from build123d import *

# Parameters (mm, degrees)
F0_W     = 20
F0_H     = 12
F1_DEPTH = 6
F2_R     = 1.6175230868
F4_DEPTH = 0.3
F5_W     = 9.6640973352
F5_H     = 2.0774973091
F6_DEPTH = 0.1
F8_DEPTH = 25


with BuildPart() as f1:
    # F0 (on Top) → F1 (new body)
    with BuildSketch(Plane.XY):
        Rectangle(F0_W, F0_H)
    extrude(amount=F1_DEPTH)

    # F2
    f2_edges = [f1.edges().sort_by_distance(p)[0] for p in [
        (10, 0, 6),
        (-10, 0, 6),
    ]]
    fillet(f2_edges, radius=F2_R)

    # F3 (on face) → F4 (join)
    with BuildSketch(Plane(origin=(0, 6, 0), x_dir=(-1, 0, 0), z_dir=(0, 1, 0))):
        with BuildLine():
            add(Edge.make_bspline(
                [(-5.9889552958, 4.3307738066), (-6.7707574457, 5.2428768765), (-7.1497281936, 4.126935614), (-7.5286989414, 3.0109943515), (-6.3679260436, 3.2148325442), (-5.2071531458, 3.4186707368), (-5.9889552958, 4.3307738066)],
                knots=[4.7123889804, 4.7123889804, 4.7123889804, 6.8067840828, 6.8067840828, 8.9011791852, 8.9011791852, 10.9955742876, 10.9955742876, 10.9955742876], degree=2, weights=[1, 0.5, 1, 0.5, 1, 0.5, 1]))
        make_face()
        Polygon((-7.1114664897, 3.8173154462), (-6.1345444992, 4.4055692852), (-6.2445141857, 3.376125358), align=None, mode=Mode.SUBTRACT)
        with BuildLine():
            add(Edge.make_bspline(
                [(5.9889552958, 4.3307738066), (5.2071531458, 3.4186707368), (6.3679260436, 3.2148325442), (7.5286989414, 3.0109943515), (7.1497281936, 4.126935614), (6.7707574457, 5.2428768765), (5.9889552958, 4.3307738066)],
                knots=[4.7123889804, 4.7123889804, 4.7123889804, 6.8067840828, 6.8067840828, 8.9011791852, 8.9011791852, 10.9955742876, 10.9955742876, 10.9955742876], degree=2, weights=[1, 0.5, 1, 0.5, 1, 0.5, 1]))
        make_face()
        Polygon((6.1345444992, 4.4055692852), (7.1114664897, 3.8173154462), (6.2445141857, 3.376125358), align=None, mode=Mode.SUBTRACT)
    extrude(amount=F4_DEPTH)

    # F5 (on face) → F6 (join)
    with BuildSketch(Plane(origin=(0, 6, 0), x_dir=(-1, 0, 0), z_dir=(0, 1, 0))):
        with Locations((-0.4735698458, 1.9353075186)):
            Rectangle(F5_W, F5_H)
        Polygon((-5.069738923, 1.1018711375), (-5.069738923, 2.8125192574), (-4.8855133355, 2.8125192574), (-3.3977353226, 2.8125192574), (-3.2135097351, 2.8125192574), (-1.7257317222, 2.8125192574), (-1.5415061347, 2.8125192574), (-0.0537281219, 2.8125192574), (0.1304974656, 2.8125192574), (1.6182754785, 2.8125192574), (1.802501066, 2.8125192574), (3.2902790789, 2.8125192574), (3.4745046664, 2.8125192574), (4.1262808791, 2.8125192574), (4.1262808791, 1.4788382144), (4.1262808791, 1.1018711375), (2.6385028662, 1.1018711375), (2.4542772787, 1.1018711375), (0.9664992658, 1.1018711375), (0.7822736783, 1.1018711375), (-0.7055043345, 1.1018711375), (-0.889729922, 1.1018711375), (-2.3775079349, 1.1018711375), (-2.5617335224, 1.1018711375), (-4.0495115353, 1.1018711375), (-4.2337371228, 1.1018711375), align=None, mode=Mode.SUBTRACT)
        Polygon((-4.8855133355, 2.8125192574), (-5.069738923, 2.8125192574), (-4.2337371228, 1.1018711375), (-4.141624329, 1.2903546759), align=None)
        Polygon((-3.3056225288, 2.624035719), (-3.3977353226, 2.8125192574), (-4.141624329, 1.2903546759), (-4.0495115353, 1.1018711375), align=None)
        Polygon((-2.4696207287, 1.2903546759), (-3.2135097351, 2.8125192574), (-3.3056225288, 2.624035719), (-2.5617335224, 1.1018711375), align=None)
        Polygon((-1.6336189285, 2.624035719), (-1.7257317222, 2.8125192574), (-2.4696207287, 1.2903546759), (-2.3775079349, 1.1018711375), align=None)
        Polygon((-0.7976171283, 1.2903546759), (-1.5415061347, 2.8125192574), (-1.6336189285, 2.624035719), (-0.889729922, 1.1018711375), align=None)
        Polygon((0.0383846719, 2.624035719), (-0.0537281219, 2.8125192574), (-0.7976171283, 1.2903546759), (-0.7055043345, 1.1018711375), align=None)
        Polygon((0.8743864721, 1.2903546759), (0.1304974656, 2.8125192574), (0.0383846719, 2.624035719), (0.7822736783, 1.1018711375), align=None)
        Polygon((1.7103882723, 2.624035719), (1.6182754785, 2.8125192574), (0.8743864721, 1.2903546759), (0.9664992658, 1.1018711375), align=None)
        Polygon((2.5463900724, 1.2903546759), (1.802501066, 2.8125192574), (1.7103882723, 2.624035719), (2.4542772787, 1.1018711375), align=None)
        Polygon((3.3823918726, 2.624035719), (3.2902790789, 2.8125192574), (2.5463900724, 1.2903546759), (2.6385028662, 1.1018711375), align=None)
        Polygon((4.1262808791, 1.4788382144), (3.4745046664, 2.8125192574), (3.3823918726, 2.624035719), (4.1262808791, 1.1018711375), align=None)
        Polygon((-4.141624329, 1.2903546759), (-4.2337371228, 1.1018711375), (-4.0495115353, 1.1018711375), align=None)
        Polygon((-3.2135097351, 2.8125192574), (-3.3977353226, 2.8125192574), (-3.3056225288, 2.624035719), align=None)
        Polygon((-2.4696207287, 1.2903546759), (-2.5617335224, 1.1018711375), (-2.3775079349, 1.1018711375), align=None)
        Polygon((-1.5415061347, 2.8125192574), (-1.7257317222, 2.8125192574), (-1.6336189285, 2.624035719), align=None)
        Polygon((-0.7976171283, 1.2903546759), (-0.889729922, 1.1018711375), (-0.7055043345, 1.1018711375), align=None)
        Polygon((0.1304974656, 2.8125192574), (-0.0537281219, 2.8125192574), (0.0383846719, 2.624035719), align=None)
        Polygon((0.8743864721, 1.2903546759), (0.7822736783, 1.1018711375), (0.9664992658, 1.1018711375), align=None)
        Polygon((1.802501066, 2.8125192574), (1.6182754785, 2.8125192574), (1.7103882723, 2.624035719), align=None)
        Polygon((2.5463900724, 1.2903546759), (2.4542772787, 1.1018711375), (2.6385028662, 1.1018711375), align=None)
        Polygon((3.4745046664, 2.8125192574), (3.2902790789, 2.8125192574), (3.3823918726, 2.624035719), align=None)
    extrude(amount=F6_DEPTH)

    # F7 (on face) → F8 (cut)
    with BuildSketch(Plane.YZ.offset(10)):
        with BuildLine():
            add(Edge.make_bspline(
                [(-2.6326957159, 0), (-1.952913386, 0.6265651125), (-1.0674622337, 0.7346938286), (-0.1766542916, 0.661617056), (0.5543848965, 0)],
                knots=[0, 0, 0, 0, 0.4953425033, 1, 1, 1, 1], degree=3))
            Line((-2.6326957159, 0), (0.5543848965, 0))
        make_face()
    extrude(amount=-F8_DEPTH, mode=Mode.SUBTRACT)


solid = f1.part
The model under review builds one solid part; all positions refer to its coordinate system, in mm. A direction names the side the tool comes from. Give positions to 0.01 mm unless a question says otherwise; leave off trailing zeros. Write item = value, one per line. Start each with the question number.
(1) Tool access review of faces 1 (the flat face through (-10, 0, 2)), 2 (the flat face through (0.8, 6, 2.2)): name each direction out of +Z, -Z, +X, -X, +Y, -Y from which nothing blocks a thin tool from reaching the whole face with its end or side.
(2) For pin 1 Ø1.5 at (x, z) = (4.5, 1.5) entering from +Y; pin 2 Ø1 at (y, z) = (-3, 5) entering from +X, all flat-tipped, find the tip position at first contact; note any pin that passes through.
(3) Draft analysis for pull direction Z (two halves, no side actions). For faces 3 (the cylindrical face through (-9.54, 0.08, 5.51)), 4 (the flat face through (0, -4, 0)), 5 (the flat face through (0, -6, 3)), 6 (the flat face through (1.6, 6, 1.7)), state which applies: +Z half, -Z half, draft (parallel to the pull), parting line (faces both ways), or undercut.
(4) For L1, parallel to X at y = 1.5, z = 4.5; L2, parallel to Y at x = 5.5, z = 3.5; L3, parallel to Z at x = -6.75, y = 6.25, list the stretches that pass through material, from the lowest coordinate up. Write a range as from..to.
Returned:
q1.face_1 = +Z, -Z, -X, +Y, -Y
q1.face_2 = +Y
q2.pin_1 = 6.1
q2.pin_2 = 10
q3.face_3 = +Z half
q3.face_4 = -Z half
q3.face_5 = draft
q3.face_6 = undercut
q4.L1 = -10..10
q4.L2 = -6..6
q4.L3 = 3.26..3.63, 4.03..4.54
